Can you work these out from the model? Positions are in its coordinate system, mm. Give positions to 0.01 mm unless a question says otherwise; leave off trailing zeros. Write each loop counter-clockwise with the first axis right and the second up, starting at its lowest first coordinate (ties: lowest second). Pieces come first, ordered by that corner, then holes.
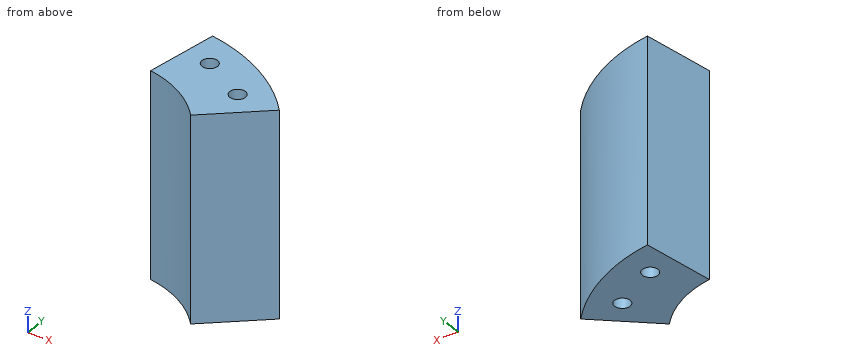
from build123d import *

# Parameters (mm, degrees)
CYLINDER222_R               = 1.5
CYLINDER222_DEPTH           = 60
CYLINDER221_R               = 1.5
CYLINDER221_DEPTH           = 60
COMPOUND199_PLACEMENT_ANGLE = 60
BOX092_W                    = 50
BOX092_H                    = 50
BOX092_DEPTH                = 39
BOX092_PLACEMENT_ANGLE      = 80
BOX093_W                    = 50
BOX093_H                    = 50
BOX093_DEPTH                = 39
BOX093_PLACEMENT_ANGLE      = 50
BOX095_W                    = 50
BOX095_H                    = 100
BOX095_DEPTH                = 39
BOX095_PLACEMENT_ANGLE      = 150
BOX094_W                    = 50
BOX094_H                    = 100
BOX094_DEPTH                = 39
BOX094_PLACEMENT_ANGLE      = 240
TUBE017_R                   = 35
TUBE017_R_2                 = 21
TUBE017_DEPTH               = 39


with BuildPart() as obj1:
    # Cylinder222 → Cylinder222 (new body)
    with BuildSketch(Plane(origin=(29, -5, -6), x_dir=(1, 0, 0), z_dir=(0, 0, 1))):
        Circle(CYLINDER222_R)
    extrude(amount=CYLINDER222_DEPTH)


with BuildPart() as compound199:
    # Cylinder221 → Cylinder221 (new body)
    with BuildSketch(Plane(origin=(29, 5, -6), x_dir=(1, 0, 0), z_dir=(0, 0, 1))):
        Circle(CYLINDER221_R)
    extrude(amount=CYLINDER221_DEPTH)

    # Compound199: union obj1
    add(obj1.part)


with BuildPart() as compound199_1:
    # Compound199 placement: moved
    add(compound199.part.rotate(Axis((0, 0, 0), (0, 0, 1)), COMPOUND199_PLACEMENT_ANGLE))


with BuildPart() as krychle092:
    # Box092 → Box092 (new body)
    with BuildSketch(Plane.XY):
        with Locations((25, 25)):
            Rectangle(BOX092_W, BOX092_H)
    extrude(amount=BOX092_DEPTH)


with BuildPart() as krychle092_1:
    # Box092 placement: moved
    add(krychle092.part.moved(Location((0, 0, 8))).rotate(Axis((0, 0, 8), (0, 0, 1)), BOX092_PLACEMENT_ANGLE))


with BuildPart() as krychle093:
    # Box093 → Box093 (new body)
    with BuildSketch(Plane.XY):
        with Locations((25, 25)):
            Rectangle(BOX093_W, BOX093_H)
    extrude(amount=BOX093_DEPTH)


with BuildPart() as krychle093_1:
    # Box093 placement: moved
    add(krychle093.part.moved(Location((0, 0, 8))).rotate(Axis((0, 0, 8), (0, 0, -1)), BOX093_PLACEMENT_ANGLE))


with BuildPart() as krychle095:
    # Box095 → Box095 (new body)
    with BuildSketch(Plane.XY):
        with Locations((25, 50)):
            Rectangle(BOX095_W, BOX095_H)
    extrude(amount=BOX095_DEPTH)


with BuildPart() as krychle095_1:
    # Box095 placement: moved
    add(krychle095.part.moved(Location((0, 0, 8))).rotate(Axis((0, 0, 8), (0, 0, 1)), BOX095_PLACEMENT_ANGLE))


with BuildPart() as krychle094:
    # Box094 → Box094 (new body)
    with BuildSketch(Plane.XY):
        with Locations((25, 50)):
            Rectangle(BOX094_W, BOX094_H)
    extrude(amount=BOX094_DEPTH)


with BuildPart() as krychle094_1:
    # Box094 placement: moved
    add(krychle094.part.moved(Location((0, 0, 8))).rotate(Axis((0, 0, 8), (0, 0, 1)), BOX094_PLACEMENT_ANGLE))


with BuildPart() as cut106:
    # Tube017 → Tube017 (new body)
    with BuildSketch(Plane.XY.offset(8)):
        Circle(TUBE017_R)
        Circle(TUBE017_R_2, mode=Mode.SUBTRACT)
    extrude(amount=TUBE017_DEPTH)

    # Cut102: cut Krychle094
    add(krychle094_1.part, mode=Mode.SUBTRACT)

    # Cut103: cut Krychle095
    add(krychle095_1.part, mode=Mode.SUBTRACT)

    # Cut104: cut Krychle093
    add(krychle093_1.part, mode=Mode.SUBTRACT)

    # Cut105: cut Krychle092
    add(krychle092_1.part, mode=Mode.SUBTRACT)

    # Cut106: cut Compound199
    add(compound199_1.part, mode=Mode.SUBTRACT)


solid = cut106.part
(1) Imagine slicing it at C-C, the plane x = 14.75. Write out the boundary of the cut face in (y, z).
Returned:
outline: (14.95, 8) - (31.74, 8) - (31.74, 47) - (14.95, 47) - close
(2) Will these pins go through, and if not, where does the flat tip stop? P1, Ø1.8, axis at x = 10.17, y = 27.61, coming from the +Z side; P2, Ø5, axis at y = 22, z = 25, coming from the +X side; P3, Ø3, axis at y = 27, z = 30.5, coming from the +X side; P4, Ø12, axis at x = 20, z = 15.5, coming from the -Y side.
Returned:
P1: passes through
P2: stops at x = 26.81
P3: stops at x = 23.97
P4: stops at y = 13.5
(3) Imagine slicing it at D-D, the plane y = 30.5. Write out the boundary of the cut face in (x, z), plus the area to 3 significant figures.
Returned:
outline: (5.38, 8) - (17.17, 8) - (17.17, 47) - (5.38, 47) - close
area: 460 mm2
(4) If I drill on L1, parallel to X at y = 23.5, z = 39.5; L2, parallel to Y at x = 10.75, z = 20.5; L3, parallel to Y at x = 11, z = 27.5, over which ranges is the centre line in solid material (lowest first)?
Returned:
L1: x = 4.14 to 17.62, 20.04 to 25.94
L2: y = 18.04 to 26.23, 29 to 33.31
L3: y = 17.89 to 26.37, 28.86 to 33.23
(5) Imagine slicing it at B-B, the plane z = 19. Write out the boundary of the cut face in (x, y), plus the area to 3 significant figures.
Returned:
outline: (3.65, 20.68) arc R21 cw to (16.09, 13.5) - (26.81, 22.5) arc R35 ccw to (6.08, 34.47) - close; hole circle Ø3 at (10.17, 27.61); hole circle Ø3 at (18.83, 22.61)
area: 260 mm2
(6) Imagine slicing it at A-A, the plane y = 27.5. Write out the boundary of the cut face in (x, z).
Returned:
outline: (4.85, 8) - (8.67, 8) - (8.67, 47) - (4.85, 47) - close; (11.67, 8) - (21.65, 8) - (21.65, 47) - (11.67, 47) - close
